Check sheet for the modelled part. Datum: model origin and axes. Units: mm. Face numbers are marked on the shaded views. A direction names the side the tool comes from. Round coordinates to 2 decimals unless told otherwise and drop trailing zeros. Write each loop counter-clockwise with the first axis right and the second up, starting at its lowest first coordinate (ties: lowest second). Pieces come first, ordered by that corner, then holes.
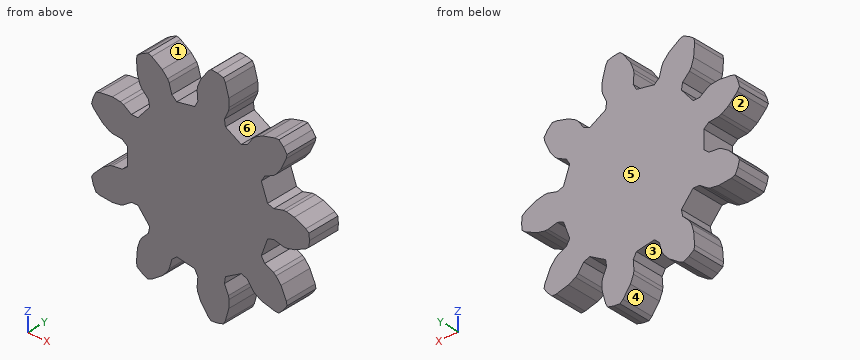
from build123d import *

# Parameters (mm, degrees)
F1_DEPTH = 6.83


with BuildPart() as f1:
    # F0 (on Front) → F1 (new body)
    with BuildSketch(Plane.XZ):
        Polygon((15.519771, -15.867663), (16.363313, -15.884129), (17.291792, -14.95565), (18.044936, -13.880049), (17.882241, -13.052181), (16.783051, -10.634822), (15.756368, -9.310512), (15.214718, -8.873741), (13.389754, -8.001385), (12.684403, -6.833367), (13.984836, -3.260458), (15.275953, -2.819095), (17.234696, -3.323895), (17.930376, -3.337475), (19.568111, -2.982934), (21.963987, -1.837675), (22.620762, -1.30807), (22.735203, 0), (22.620762, 1.30807), (21.963987, 1.837675), (19.568111, 2.982934), (17.930376, 3.337475), (17.234696, 3.323895), (15.275953, 2.819095), (13.984836, 3.260458), (12.684403, 6.833367), (13.389754, 8.001385), (15.214718, 8.873741), (15.756368, 9.310512), (16.783051, 10.634822), (17.882241, 13.052181), (18.044936, 13.880049), (17.291792, 14.95565), (16.363313, 15.884129), (15.519771, 15.867663), (12.948265, 15.204942), (11.465793, 14.423821), (10.9416, 13.966244), (9.765596, 12.320488), (8.49284, 11.828678), (5.200029, 13.729783), (4.989571, 15.077928), (5.826835, 16.919255), (5.961012, 17.602008), (5.896247, 19.276427), (5.184426, 21.834777), (4.776915, 22.573538), (3.50859, 22.913385), (2.20052, 23.027827), (1.564913, 22.472995), (0.021014, 20.312389), (-0.612531, 18.761101), (-0.719961, 18.073632), (-0.562961, 16.056989), (-1.221819, 14.862128), (-4.966266, 14.201881), (-5.994056, 15.09934), (-6.536257, 17.048062), (-6.872337, 17.657328), (-7.998246, 18.898377), (-10.188008, 20.400638), (-10.975046, 20.704619), (-12.165089, 20.149693), (-13.24069, 19.396549), (-13.370954, 18.562963), (-13.164839, 15.915443), (-12.653013, 14.319853), (-12.293413, 13.724166), (-10.876871, 12.280246), (-10.613544, 10.941424), (-13.057558, 8.028761), (-14.421767, 8.055604), (-16.089731, 9.199891), (-16.738811, 9.450588), (-18.399039, 9.677567), (-21.042128, 9.420813), (-21.84043, 9.147778), (-22.395356, 7.957735), (-22.735202, 6.68941), (-22.299172, 5.967114), (-20.439486, 4.071485), (-19.021779, 3.178187), (-18.363409, 2.953011), (-16.350141, 2.757439), (-15.287842, 1.901105), (-15.287842, -1.901105), (-16.350141, -2.757439), (-18.363409, -2.953011), (-19.021779, -3.178187), (-20.439486, -4.071485), (-22.299172, -5.967114), (-22.735202, -6.68941), (-22.395356, -7.957735), (-21.84043, -9.147778), (-21.042128, -9.420813), (-18.399039, -9.677567), (-16.738811, -9.450588), (-16.089731, -9.199891), (-14.421767, -8.055604), (-13.057558, -8.028761), (-10.613544, -10.941424), (-10.876871, -12.280246), (-12.293413, -13.724166), (-12.653013, -14.319853), (-13.164839, -15.915443), (-13.370954, -18.562963), (-13.24069, -19.396549), (-12.165089, -20.149693), (-10.975046, -20.704619), (-10.188008, -20.400638), (-7.998246, -18.898377), (-6.872337, -17.657328), (-6.536257, -17.048062), (-5.994056, -15.09934), (-4.966266, -14.201881), (-1.221819, -14.862128), (-0.562961, -16.056989), (-0.719961, -18.073632), (-0.612531, -18.761101), (0.021014, -20.312389), (1.564913, -22.472995), (2.20052, -23.027827), (3.50859, -22.913385), (4.776915, -22.573538), (5.184426, -21.834777), (5.896247, -19.276427), (5.961012, -17.602008), (5.826835, -16.919255), (4.989571, -15.077928), (5.200029, -13.729783), (8.49284, -11.828678), (9.765596, -12.320488), (10.9416, -13.966244), (11.465793, -14.423821), (12.948265, -15.204942), align=None)
    extrude(amount=F1_DEPTH)


solid = f1.part
1. Set-up check for the marked faces 4, 5 and 6: record each of +Z, -Z, +X, -X, +Y, -Y from which the full face is reachable in a straight line by a thin tool's end or side.
2. Scan lines: line 1 along Z through (x, y) = (14.5, -6.5); line 2 along X through (y, z) = (-6.25, 15); line 3 along Z through (x, y) = (17.5, -3.75). Record each from-to range of solid material in increasing order.
3. Release check for a two-part mould opening along Z. For the marked faces 1, 2 and 3 record: released by +Z, released by -Z, zero draft, split by the parting line, or undercut.
4. Go/stop test with flat-tipped pins: pin 1 (3 mm diameter, centred on x = 14, y = -4, fed in from -Z); pin 2 (2 mm diameter, centred on y = -1, z = -18.5, fed in from +X); pin 3 (1 mm diameter, centred on x = 17.5, y = -1.5, fed in from +Z). Record where each tip stops, or that it passes through.
5. Sectioned sample at A-A, the plane x = -17.5. Enter the section's corners in (y, z).
6. Sectioned sample at B-B, the plane x = 1. Enter the section's corners in (y, z), plus the area to 3 significant figures.
Computed values:
1. face 4: -Z, +Y, -Y
1. face 5: +Z, -Z, +X, -X, +Y
1. face 6: +Y, -Y
2. line 1: z = -15.6 to -8.53, -3.08 to 3.08, 8.53 to 15.6
2. line 2: x = -12.87 to -5.88, -1.15 to 5, 12.56 to 17.25
2. line 3: z = -14.66 to -12.21, -3.33 to 3.33, 12.21 to 14.66
3. face 1: released by +Z
3. face 2: undercut
3. face 3: released by -Z
4. pin 1: stops at z = -15.86
4. pin 2: stops at x = 5.96
4. pin 3: stops at z = 15.25
5. outline: (-6.83, -9.55) - (0, -9.55) - (0, -2.87) - (-6.83, -2.87) - close; (-6.83, 2.87) - (0, 2.87) - (0, 9.55) - (-6.83, 9.55) - close
6. outline: (-6.83, -21.68) - (0, -21.68) - (0, 21.68) - (-6.83, 21.68) - close
6. area: 296 mm2
